Part model, mm, in its own coordinate system. Face numbers are marked on the shaded views. Round coordinates to 2 decimals unless told otherwise and drop trailing zeros. Write each loop counter-clockwise with the first axis right and the second up, starting at its lowest first coordinate (ties: lowest second). Pieces come first, ordered by that corner, then holes. Notation, with made-up numbers: M 87,21.25 L 126,21.25 A30 cw 126,53.25 Z; hole C 87.25,18.5 d11. An arc over 180 degrees is marked long. Answer as a JSON object with one key per item and string values. Group by question number.
1. Drill centre lines: line 1 (Z direction, x = 3.75, y = 59); line 2 (Y direction, x = 11.25, z = 29); line 3 (Y direction, x = 4, z = 27). Where is each one in solid material? Low to high. Write a range as from..to.
2. Band-saw the part on A-A, the plane y = -18. Write the cut outline in (x, z), plus the area to 3 significant figures.
3. Drop flat-ended pins along their axis: pin 1 (2.5 mm diameter, centred on y = -79, z = -101.5, fed in from -X); pin 2 (2.5 mm diameter, centred on y = -71, z = -102.5, fed in from +X). Give the stop position or say it passes through.
4. Two-plate mould, pull along X, no slides. Class the marked faces 1 and 2: +X half, -X half, draft (parallel to the pull), parting line (faces both ways), or undercut.
from build123d import *

# Parameters (mm, degrees)
F0_W     = 370
F0_H     = 150
F0_R     = 5
F1_DEPTH = 10
F2_W     = 370
F2_H     = 5
F3_DEPTH = 5


with BuildPart() as f1:
    # F0 (on Right) → F1 (new body)
    with BuildSketch(Plane.YZ):
        with Locations((-14.059471, -33.810468)):
            Rectangle(F0_W, F0_H)
        with Locations((-125.059471, 28.689532)):
            Circle(F0_R, mode=Mode.SUBTRACT)
        with Locations((-51.059471, 28.689532)):
            Circle(F0_R, mode=Mode.SUBTRACT)
        with Locations((22.940529, 28.689532)):
            Circle(F0_R, mode=Mode.SUBTRACT)
        with Locations((96.940529, 28.689532)):
            Circle(F0_R, mode=Mode.SUBTRACT)
    extrude(amount=F1_DEPTH)

    # F2 (on face) → F3 (cut)
    with BuildSketch(Plane(origin=(0, 0, 0), x_dir=(0, -1, 0), z_dir=(-1, 0, 0))):
        with Locations((14.059471, -101.310468)):
            Rectangle(F2_W, F2_H)
    extrude(amount=-F3_DEPTH, mode=Mode.SUBTRACT)

    # F4: F1 across face


with BuildPart() as f1_1:
    add(f1.part)
    add(f1.part.mirror(Plane(origin=(10, -14.059471, -34.166265), x_dir=(0, 1, 0), z_dir=(1, 0, 0))))


solid = f1_1.part
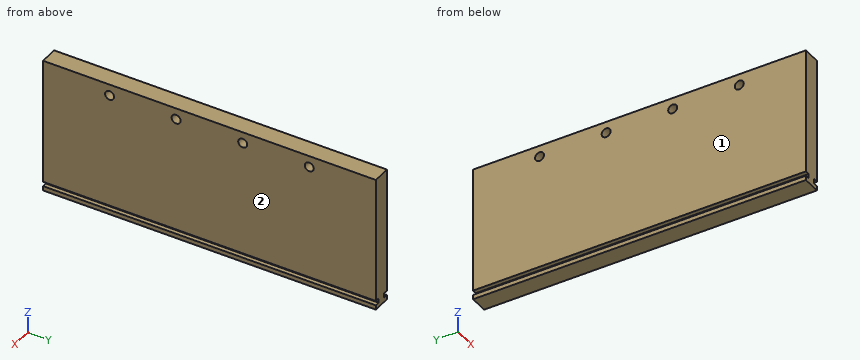
Worked answers:
{
 "1": {"line 1": "z = -108.81..-103.81, -98.81..41.19", "line 2": "y = -199.06..-130.05, -120.07..-56.05, -46.07..17.95, 27.93..91.95, 101.93..170.94", "line 3": "y = -199.06..-129.77, -120.35..-55.77, -46.35..18.23, 27.65..92.23, 101.65..170.94"},
 "2": {"outline": "M 0,-108.81 L 20,-108.81 L 20,-103.81 L 15,-103.81 L 15,-98.81 L 20,-98.81 L 20,41.19 L 0,41.19 L 0,-98.81 L 5,-98.81 L 5,-103.81 L 0,-103.81 Z", "area": "2,950 mm^2"},
 "3": {"pin 1": "stops at x = 5", "pin 2": "stops at x = 15"},
 "4": {"face 1": "-X half", "face 2": "+X half"}
}
